Work out the finished part from the listing and answer in its coordinate system (mm). A direction names the side the tool comes from. Round coordinates to 2 decimals unless told otherwise and drop trailing zeros. Write each loop counter-clockwise with the first axis right and the second up, starting at its lowest first coordinate (ties: lowest second). Pieces come first, ordered by that corner, then holes. Notation, with made-up numbers: (-16, 17.5) -> (34, 17.5) arc R32 cw to (34, 46.5) -> close; hole circle Ø2 at (76.5, -4). An arc over 180 degrees is marked (long way). One line per item, written item: value.
```python
from build123d import *

# Parameters (mm, degrees)
SKETCH_R             = 15
SKETCH_R_2           = 1.5
PAD_DEPTH            = 3
SKETCH002_R          = 2.25
POCKET_DEPTH         = 2
SKETCH001_R          = 5
POCKET001_DEPTH      = 1
SKETCH003_R          = 2.5
POCKET002_DEPTH      = 2
POCKET002_FACE17_R   = 5
POCKET002_FACE17_R_2 = 2.25
PAD001_DEPTH         = 1
CHAMFER_SIZE         = 0.4
CHAMFER001_SIZE      = 0.5
CHAMFER002_SIZE      = 0.4
CHAMFER003_SIZE      = 0.5


with BuildPart() as part:
    # Sketch → Pad (new body)
    with BuildSketch(Plane.XY):
        Circle(SKETCH_R)
        with Locations((0, 11)):
            Circle(SKETCH_R_2, mode=Mode.SUBTRACT)
        with Locations((-11, 0)):
            Circle(SKETCH_R_2, mode=Mode.SUBTRACT)
        with Locations((0, -11)):
            Circle(SKETCH_R_2, mode=Mode.SUBTRACT)
        with Locations((11, 0)):
            Circle(SKETCH_R_2, mode=Mode.SUBTRACT)
    extrude(amount=PAD_DEPTH)

    # Sketch002 (on Face7 of Pad) → Pocket (cut)
    with BuildSketch(Plane.XY.offset(3)):
        Circle(SKETCH002_R)
    extrude(amount=-POCKET_DEPTH, mode=Mode.SUBTRACT)

    # Sketch001 (on Face7 of Pad) → Pocket001 (cut)
    with BuildSketch(Plane.XY.offset(3)):
        Circle(SKETCH001_R)
    extrude(amount=-POCKET001_DEPTH, mode=Mode.SUBTRACT)

    # Sketch003 (on Face2 of Pocket001) → Pocket002 (cut)
    with BuildSketch(Plane(origin=(0, 0, 0), x_dir=(1, 0, 0), z_dir=(0, 0, -1))):
        with Locations((0, 11)):
            Circle(SKETCH003_R)
        with Locations((11, 0)):
            Circle(SKETCH003_R)
        with Locations((0, -11)):
            Circle(SKETCH003_R)
        with Locations((-11, 0)):
            Circle(SKETCH003_R)
    extrude(amount=-POCKET002_DEPTH, mode=Mode.SUBTRACT)

    # Pocket002 Face17 → Pad001 (add)
    with BuildSketch(Plane(origin=(0, 0, 2), x_dir=(0, 1, 0), z_dir=(0, 0, 1))):
        Circle(POCKET002_FACE17_R)
        Circle(POCKET002_FACE17_R_2, mode=Mode.SUBTRACT)
    extrude(amount=PAD001_DEPTH)

    # Chamfer
    chamfer_edges = [part.edges().sort_by_distance(p)[0] for p in [
        (-1.5, -11, 3),
        (-12.5, 0, 3),
        (-1.5, 11, 3),
        (9.5, 0, 3),
    ]]
    chamfer(chamfer_edges, length=CHAMFER_SIZE)

    # Chamfer001
    chamfer001_edges = [part.edges().sort_by_distance(p)[0] for p in [
        (-2.25, 0, 3),
    ]]
    chamfer(chamfer001_edges, length=CHAMFER001_SIZE)

    # Chamfer002
    chamfer002_edges = [part.edges().sort_by_distance(p)[0] for p in [
        (9.5, 0, 2),
        (-1.5, -11, 2),
        (-12.5, 0, 2),
        (-1.5, 11, 2),
    ]]
    chamfer(chamfer002_edges, length=CHAMFER002_SIZE)

    # Chamfer003
    chamfer003_edges = [part.edges().sort_by_distance(p)[0] for p in [
        (-2.5, -11, 0),
        (8.5, 0, 0),
        (-13.5, 0, 0),
        (-2.5, 11, 0),
    ]]
    chamfer(chamfer003_edges, length=CHAMFER003_SIZE)


solid = part.part
```
(1) Find section A-A on x = 11. Give the vertices of the cut face in (y, z).
Reported:
outline: (-10.2, 0) -> (-3, 0) -> (-2.5, 0.5) -> (-2.5, 2) -> (-1.9, 2) -> (-1.5, 2.4) -> (-1.5, 2.6) -> (-1.9, 3) -> (-10.2, 3) -> close; (1.5, 2.4) -> (1.9, 2) -> (2.5, 2) -> (2.5, 0.5) -> (3, 0) -> (10.2, 0) -> (10.2, 3) -> (1.9, 3) -> (1.5, 2.6) -> close
(2) Flat-ended cylindrical pins translate along their axes: pin 1 Ø2 at (x, y) = (0, 1) entering from +Z; pin 2 Ø2.5 at (x, y) = (1, 10.5) entering from -Z; pin 3 Ø1.8 at (x, y) = (0, 11) entering from -Z; pin 4 Ø1.5 at (x, z) = (-3, 2.5) entering from +Y. Find the tip coordinate at first contact, or state that the pin passes through.
Reported:
pin 1: stops at z = 1
pin 2: stops at z = 2
pin 3: passes through
pin 4: stops at y = 14.83
(3) Consider probe 1 along Y at (x, z) = (0, 1.6); probe 2 along Y at (x, z) = (0, 2.55); probe 3 along X at (y, z) = (-0.75, 1.9). Determine where each line is inside the solid, lowest interval first.
Reported:
probe 1: y = -15 to -13.5, -8.5 to -2.25, 2.25 to 8.5, 13.5 to 15
probe 2: y = -15 to -12.5, -9.5 to -2.3, 2.3 to 9.5, 12.5 to 15
probe 3: x = -14.98 to -13.38, -8.62 to -2.12, 2.12 to 8.62, 13.38 to 14.98
(4) A tool of negligible diameter and unlimited length cuts with its end or side. For faces 1 (the face through (-14.985, 0.66, 1.479)), 2 (the face through (2, 10, 2)), from which of +Z, -Z, +X, -X, +Y, -Y can it reach the whole face along a straight path? Write none if from no direction.
Reported:
face 1: +Z, -Z
face 2: -Z
(5) Find section C-C on x = 0. Give the number of separate pieces and of enclosed holes in the cut face, plus the area to 3 significant figures.
Reported:
separate pieces: 3
enclosed holes: 0
area: 53.6 mm2
